```python
from build123d import *

# Parameters (mm, degrees)
SKETCH1_W                                  = 140
SKETCH1_H                                  = 100
BOSS_EXTRUDE1_DEPTH                        = 2
CUT_EXTRUDE2_REACH                         = 88.046
SKETCH2_R                                  = 2.515
FILLET1_R                                  = 10
MIRROR1_AT_THE_SECOND_PLANE_COPY_1_REACH   = 88.046
MIRROR1_AT_THE_SECOND_PLANE_COPY_1_SKETC_R = 2.515


with BuildPart() as part:
    # Sketch1 → Boss-Extrude1 (new body)
    with BuildSketch(Plane.XY):
        Rectangle(SKETCH1_W, SKETCH1_H)
    extrude(amount=BOSS_EXTRUDE1_DEPTH)

    # Sketch2 → Cut-Extrude2 (cut, up to next)
    with BuildSketch(Plane.XY, mode=Mode.PRIVATE) as cut_extrude2_sk1:
        with Locations(Location((-50, 31.25, 0), (0, 0, 180))):
            Circle(SKETCH2_R)
    cut_extrude2_tool1 = extrude(cut_extrude2_sk1.sketch, amount=CUT_EXTRUDE2_REACH, mode=Mode.PRIVATE) & part.part
    cut_extrude2 = cut_extrude2_tool1.solids().sort_by_distance((-50, 31.25, 0))[0]
    add(cut_extrude2, mode=Mode.SUBTRACT)

    # Fillet1
    fillet1_edges = [part.edges().sort_by_distance(p)[0] for p in [
        (70, -50, 1),
        (-70, -50, 1),
        (-70, 50, 1),
        (70, 50, 1),
    ]]
    fillet(fillet1_edges, radius=FILLET1_R)

    # Mirror1: Cut-Extrude2 across plane
    add(cut_extrude2.mirror(Plane.ZX), mode=Mode.SUBTRACT)

    # Mirror1 at the second plane: Cut-Extrude2 across plane
    add(cut_extrude2.mirror(Plane(origin=(0, 0, 0), x_dir=(0, 0, 1), z_dir=(1, 0, 0))), mode=Mode.SUBTRACT)

    # Mirror1 at the second plane copy 1 sketc → Mirror1 at the second plane copy 1 (cut, up to next)
    with BuildSketch(Plane(origin=(0, 0, 0), x_dir=(-1, 0, 0), z_dir=(0, 0, 1)), mode=Mode.PRIVATE) as mirror1_at_the_second_plane_copy_1_sk1:
        with Locations(Location((-50, 31.25, 0), (0, 0, 180))):
            Circle(MIRROR1_AT_THE_SECOND_PLANE_COPY_1_SKETC_R)
    mirror1_at_the_second_plane_copy_1_tool1 = extrude(mirror1_at_the_second_plane_copy_1_sk1.sketch, amount=MIRROR1_AT_THE_SECOND_PLANE_COPY_1_REACH, mode=Mode.PRIVATE) & part.part
    add(mirror1_at_the_second_plane_copy_1_tool1.solids().sort_by_distance((50, -31.25, 0))[0], mode=Mode.SUBTRACT)


solid = part.part
```
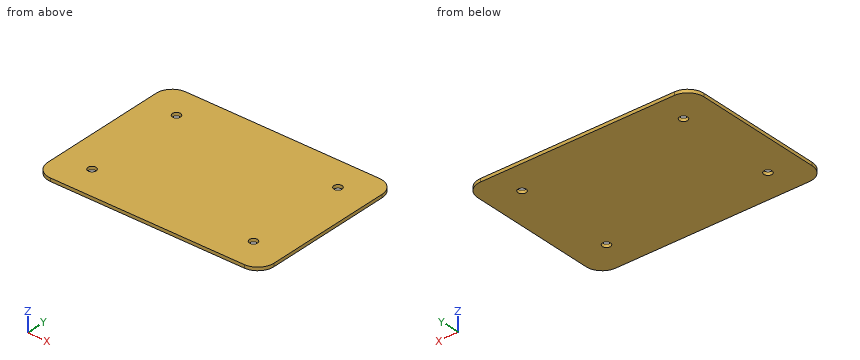
Could you check a few things on this model? Use its own coordinates, in mm. Round coordinates to 2 decimals unless told otherwise and drop trailing zeros. Loops run counter-clockwise (first coordinate to the right, second up) from the corner with the lowest first, then second, coordinate; pieces in that order, holes last. Notation, with made-up numbers: (7.5, 11) - (45.5, 11) arc R12 cw to (45.5, 30) - close; hole circle Ø5 at (5, 21.25). An arc over 180 degrees is marked (long way). Use CSV: the item, a comma, the result in double quotes.
Item 1: Will these pins go through, and if not, where does the flat tip stop? pin 1 (4 mm diameter, centred on x = 50, y = -31.25, fed in from +Z); pin 2 (8 mm diameter, centred on x = -50, y = 31.25, fed in from -Z).
Here are the results:
pin 1,"passes through"
pin 2,"stops at z = 0"
Item 2: If we section it at B-B on x = -50: List the corners of the cut face in (y, z) for me (3 decimals), then the cut area to 3 significant figures.
Here are the results:
outline,"(-50, 0) - (-33.765, 0) - (-33.765, 2) - (-50, 2) - close; (-28.735, 0) - (28.735, 0) - (28.735, 2) - (-28.735, 2) - close; (33.765, 0) - (50, 0) - (50, 2) - (33.765, 2) - close"
area,"180 mm²"
Item 3: I need wall thicknesses on L1, parallel to Y at x = -50, z = 0.6 (3 decimals); L2, parallel to X at y = 31.25, z = 0.4 (3 decimals); L3, parallel to X at y = 33, z = 0.15. Which ranges of each line are inside material? Lowest first, please. Write a range as [from, to].
Here are the results:
L1,"y = [-50, -33.765], [-28.735, 28.735], [33.765, 50]"
L2,"x = [-70, -52.515], [-47.485, 47.485], [52.515, 70]"
L3,"x = [-70, -51.81], [-48.19, 48.19], [51.81, 70]"
Item 4: If we section it at A-A on y = 31.25: List the corners of the cut face in (x, z) for me (3 decimals), then the cut area to 3 significant figures.
Here are the results:
outline,"(-70, 0) - (-52.515, 0) - (-52.515, 2) - (-70, 2) - close; (-47.485, 0) - (47.485, 0) - (47.485, 2) - (-47.485, 2) - close; (52.515, 0) - (70, 0) - (70, 2) - (52.515, 2) - close"
area,"260 mm²"
